Source: CAD feature listing. Evaluate the final solid. Frame: model axes, mm. A direction names the side the tool comes from. Round coordinates to 2 decimals unless told otherwise and drop trailing zeros. Loops run counter-clockwise (first coordinate to the right, second up) from the corner with the lowest first, then second, coordinate; pieces in that order, holes last. Notation, with made-up numbers: (-7.75, 79) - (12.25, 79) arc R27 ccw to (12.25, 108) - close; hole circle Ø6 at (42, 55). An arc over 180 degrees is marked (long way). Write item = value, one per line. Start each with the question number.
from build123d import *

# Parameters (mm, degrees)
F0_R     = 2.5
F0_R_2   = 22.5
F1_DEPTH = 2
F2_DEPTH = 4
F3_DEPTH = 49
F4_START = 2
F4_DEPTH = 2
F5_R     = 2.5
F6_R     = 1


with BuildPart() as f1:
    # F0 (on Top) → F1 (new body)
    with BuildSketch(Plane.XY):
        with BuildLine():
            ThreePointArc((-64.6104820835, -2.0913623334), (-49.905732642, -11.9825383792), (-32.9089653438, -17))
            ThreePointArc((-32.9089653438, -17), (0, -24.9371242498), (32.9089653438, -17))
            ThreePointArc((32.9089653438, -17), (49.905732642, -11.9825383792), (64.6104820835, -2.0913623334))
            Line((64.6104820835, -2.0913623334), (81.9837382259, 27.9999999982))
            Line((81.9837382291, 27.9999999928), (65.2405804184, 57))
            Line((65.2405804184, 57), (32.9089653438, 57))
            Line((32.9089653438, 57), (16.7431578065, 85))
            Line((16.7431578065, 85), (-16.7431578065, 85))
            Line((-16.7431578065, 85), (-32.9089653438, 57))
            Line((-32.9089653438, 57), (-65.2405804184, 57))
            Line((-65.2405804184, 57), (-81.9837382259, 27.9999999982))
            Line((-81.9837382259, 27.9999999982), (-64.6104820835, -2.0913623334))
        make_face()
        with Locations((-22.8121797535, -6.4300971625)):
            Circle(F0_R, mode=Mode.SUBTRACT)
        Polygon((-79.6743371482, 28), (-64.08587988, 55), (-32.9089653438, 55), (-17.3205080757, 28), (-32.9089653438, 1), (-64.08587988, 1), align=None, mode=Mode.SUBTRACT)
        with Locations((-11.5, 13)):
            Circle(F0_R, mode=Mode.SUBTRACT)
        with Locations((0, -10.200026891)):
            Circle(F0_R, mode=Mode.SUBTRACT)
        with Locations((22.8121797535, -6.4300971625)):
            Circle(F0_R, mode=Mode.SUBTRACT)
        with Locations((11.5, 13)):
            Circle(F0_R, mode=Mode.SUBTRACT)
        Polygon((64.08587988, 1), (32.9089653438, 1), (17.3205080757, 28), (32.9089653438, 55), (64.08587988, 55), (79.6743371482, 28), align=None, mode=Mode.SUBTRACT)
        Polygon((-31.1769145362, 56), (-15.5884572681, 83), (15.5884572681, 83), (31.1769145362, 56), (15.5884572681, 29), (-15.5884572681, 29), align=None, mode=Mode.SUBTRACT)
        Polygon((-32.9089653438, 55), (-64.08587988, 55), (-79.6743371482, 28), (-64.08587988, 1), (-32.9089653438, 1), (-17.3205080757, 28), align=None)
        with Locations((-48.4974226119, 28)):
            Circle(F0_R_2, mode=Mode.SUBTRACT)
        Polygon((17.3205080757, 28), (32.9089653438, 1), (64.08587988, 1), (79.6743371482, 28), (64.08587988, 55), (32.9089653438, 55), align=None)
        with Locations((48.4974226119, 28)):
            Circle(F0_R_2, mode=Mode.SUBTRACT)
    extrude(amount=F1_DEPTH)

    # F0 (on Top) → F2 (join)
    with BuildSketch(Plane.XY):
        with BuildLine():
            ThreePointArc((-64.6104820835, -2.0913623334), (-49.905732642, -11.9825383792), (-32.9089653438, -17))
            ThreePointArc((-32.9089653438, -17), (0, -24.9371242498), (32.9089653438, -17))
            ThreePointArc((32.9089653438, -17), (49.905732642, -11.9825383792), (64.6104820835, -2.0913623334))
            Line((64.6104820835, -2.0913623334), (81.9837382259, 27.9999999982))
            Line((81.9837382291, 27.9999999928), (65.2405804184, 57))
            Line((65.2405804184, 57), (32.9089653438, 57))
            Line((32.9089653438, 57), (16.7431578065, 85))
            Line((16.7431578065, 85), (-16.7431578065, 85))
            Line((-16.7431578065, 85), (-32.9089653438, 57))
            Line((-32.9089653438, 57), (-65.2405804184, 57))
            Line((-65.2405804184, 57), (-81.9837382259, 27.9999999982))
            Line((-81.9837382259, 27.9999999982), (-64.6104820835, -2.0913623334))
        make_face()
        with Locations((-22.8121797535, -6.4300971625)):
            Circle(F0_R, mode=Mode.SUBTRACT)
        Polygon((-79.6743371482, 28), (-64.08587988, 55), (-32.9089653438, 55), (-17.3205080757, 28), (-32.9089653438, 1), (-64.08587988, 1), align=None, mode=Mode.SUBTRACT)
        with Locations((-11.5, 13)):
            Circle(F0_R, mode=Mode.SUBTRACT)
        with Locations((0, -10.200026891)):
            Circle(F0_R, mode=Mode.SUBTRACT)
        with Locations((22.8121797535, -6.4300971625)):
            Circle(F0_R, mode=Mode.SUBTRACT)
        with Locations((11.5, 13)):
            Circle(F0_R, mode=Mode.SUBTRACT)
        Polygon((64.08587988, 1), (32.9089653438, 1), (17.3205080757, 28), (32.9089653438, 55), (64.08587988, 55), (79.6743371482, 28), align=None, mode=Mode.SUBTRACT)
        Polygon((-31.1769145362, 56), (-15.5884572681, 83), (15.5884572681, 83), (31.1769145362, 56), (15.5884572681, 29), (-15.5884572681, 29), align=None, mode=Mode.SUBTRACT)
    extrude(amount=F2_DEPTH)

    # F0 (on Top) → F3 (join)
    with BuildSketch(Plane.XY):
        with Locations((-11.5, 13)):
            Circle(F0_R)
        with Locations((11.5, 13)):
            Circle(F0_R)
        with Locations((-22.8121797535, -6.4300971625)):
            Circle(F0_R)
        with Locations((0, -10.200026891)):
            Circle(F0_R)
        with Locations((22.8121797535, -6.4300971625)):
            Circle(F0_R)
    extrude(amount=F3_DEPTH)

    # F0 (on Top) → F4 (join)
    with BuildSketch(Plane.XY.offset(F4_START)):
        Polygon((15.5884572681, 83), (-15.5884572681, 83), (-31.1769145362, 56), (-15.5884572681, 29), (15.5884572681, 29), (31.1769145362, 56), align=None)
        with Locations((0, 56)):
            Circle(F0_R_2, mode=Mode.SUBTRACT)
    extrude(amount=F4_DEPTH)

    # F5
    f5_edges = [f1.edges().sort_by_distance(p)[0] for p in [
        (-25.31218, -6.430097, 49),
        (-14, 13, 49),
        (9, 13, 49),
        (20.31218, -6.430097, 49),
        (-2.5, -10.200027, 49),
    ]]
    fillet(f5_edges, radius=F5_R)

    # F6
    f6_edges = [f1.edges().sort_by_distance(p)[0] for p in [
        (-73.29711, 12.954319, 4),
        (-49.905733, -11.982538, 4),
        (0, -24.937124, 4),
        (49.905733, -11.982538, 4),
        (73.29711, 12.954319, 4),
        (73.612159, 42.5, 4),
        (49.074773, 57, 4),
        (24.826062, 71, 4),
        (0, 85, 4),
        (-24.826062, 71, 4),
        (-49.074773, 57, 4),
        (-73.612159, 42.5, 4),
    ]]
    fillet(f6_edges, radius=F6_R)


solid = f1.part
(1) Material intervals for line 1 along Z through (x, y) = (-24, 19); line 2 along Y through (x, z) = (0, 2.45); line 3 along Z through (x, y) = (-8, 21), sorted ascending. Write a range as from..to.
(2) Access query for faces 5 (the face through (-24.83, 70.4, 3.71)), 6 (the face through (-12.04, 10.56, 24.95)), 7 (the face through (23.5, 42.7, 1)). Directions: +Z, -Z, +X, -X, +Y, -Y. A direction counts if a zero-diameter tool reaches every point of the face in a straight line with its end or side. Return the directions, or none.
(3) Pin query (flat end, axial travel): P1, Ø1.5, axis at x = 4.5, y = 10, coming from the -Z side; P2, Ø1, axis at x = 56, z = 3, coming from the +Y side; P3, Ø4, axis at y = 14, z = 19.5, coming from the -X side; P4, Ø3, axis at x = -3, z = 22.5, coming from the +Y side. Return the tip coordinate at first contact, or that it passes through.
(4) Mould query, pull axis X, two halves, no side actions, for faces 1 (the face through (-42, 50, 2)), 2 (the face through (-50.131, -11.876, 1.479)), 3 (the face through (7, 78, 2)), 4 (the face through (73.235, 42.553, 3.715)). Classes: +X half, -X half, draft (parallel to the pull), parting line (faces both ways), or undercut.
(5) Cut plane A-A (x = 0). Output: boundary loops of the cut face in (y, z), and give its area (3 significant figures).
(6) Cut plane B-B (z = 34). Output: boundary loops of the cut face in (x, y).
(7) Cut plane C-C (y = 13). State how many separate pieces and enclosed holes the cut face has, and give its area (3 significant figures).
Solution:
q1.line_1 = 0..2
q1.line_2 = -24.94..33.5, 78.5..85
q1.line_3 = 0..4
q2.face_5 = +Z, -X, +Y
q2.face_6 = +Z
q2.face_7 = -Z
q3.P1 = 0
q3.P2 = 57
q3.P3 = -14
q3.P4 = -8.2
q4.face_1 = undercut
q4.face_2 = -X half
q4.face_3 = undercut
q4.face_4 = +X half
q5.outline = (-24.94, 0) - (29, 0) - (29, 2) - (33.5, 2) - (33.5, 4) - (-7.7, 4) - (-7.7, 46.5) arc R2.5 ccw to (-12.7, 46.5) - (-12.7, 4) - (-23.94, 4) arc R1 ccw to (-24.94, 3) - close; (78.5, 2) - (83, 2) - (83, 0) - (85, 0) - (85, 3) arc R1 ccw to (84, 4) - (78.5, 4) - close
q5.area = 464 mm^2
q6.outline = circle Ø5 at (-22.81, -6.43); circle Ø5 at (-11.5, 13); circle Ø5 at (0, -10.2); circle Ø5 at (11.5, 13); circle Ø5 at (22.81, -6.43)
q7.separate_pieces = 3
q7.enclosed_holes = 0
q7.area = 716 mm^2
